Input: part model. Units: mm. Frame: model coordinates. Face numbers are marked on the shaded views. A direction names the side the tool comes from. Give positions to 0.01 mm unless a question says otherwise; leave off trailing zeros. Order: outer loops, then holes, each group sorted by start corner. A loop starts at its lowest first (then second) coordinate and runs counter-clockwise, first axis right, second up.
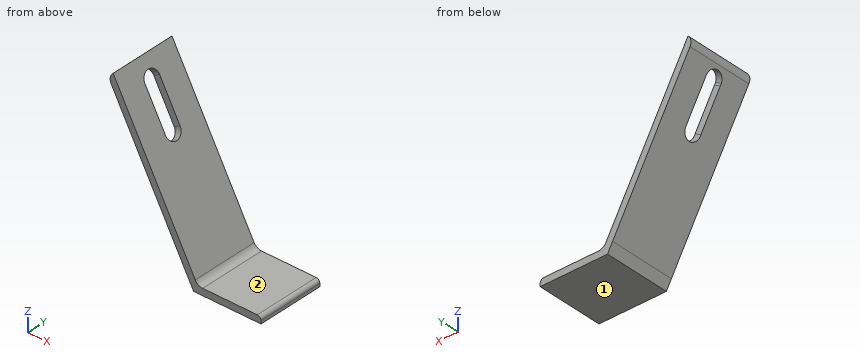
```python
from build123d import *

# Parameters (mm, degrees)
F1_DEPTH    = 40
F2_T1_DEPTH = 40
F2_T3_DEPTH = 64.4948974279
F3_T1_DEPTH = 50.8639610307
F5_DEPTH    = 25


# Not quite as in the source:
# - a fillet or chamfer that OpenCascade refuses, or shapes differently, is made with other operations: its cross-section is extruded or revolved along the edge and cut away or added
# - a feature names something its author has since deleted; it is built from what else it names


with BuildPart() as f1:
    # F0 (on Front) → F1 (new body)
    with BuildSketch(Plane.XZ):
        Polygon((-51.3135007212, 94.3231601012), (-3, 5.5145230071), (0, 0), (40, 0), (40, 4), (2.3775297152, 4), (-47.7997987259, 96.2346773752), align=None)
    extrude(amount=F1_DEPTH)

    # F2: fillet of radius 5 on 2 edges, made by hand

    # F2_s2 → F2_t1 (join)
    with BuildSketch(Plane.XZ):
        with BuildLine():
            ThreePointArc((5.3494418593, 4), (2.7947386439, 4.7019200239), (0.9573143652, 6.6106034076))
            Line((0.9573143652, 6.6106034076), (2.3775297152, 4))
            Line((2.3775297152, 4), (5.3494418593, 4))
        make_face()
    extrude(amount=F2_T1_DEPTH)

    # F2_s4 → F2_t3 (cut)
    with BuildSketch(Plane.XZ.offset(-12.2474487139)):
        with BuildLine():
            ThreePointArc((-47.7997987259, 96.2346773752), (-49.4935666702, 93.3361748844), (-48.9723797433, 90.019771603))
            Line((-48.9723797433, 90.019771603), (-51.3135007212, 94.3231601012))
            Line((-51.3135007212, 94.3231601012), (-47.7997987259, 96.2346773752))
        make_face()
    extrude(amount=F2_T3_DEPTH, mode=Mode.SUBTRACT)

    # F3: fillet of radius 2.1727922061 on 2 edges, made by hand

    # F3_s2 → F3_t1 (cut)
    with BuildSketch(Plane.XZ.offset(-5.4319805153)):
        with BuildLine():
            ThreePointArc((37.8272077939, 4), (39.3636038969, 3.3636038969), (40, 1.8272077939))
            Line((40, 1.8272077939), (40, 4))
            Line((40, 4), (37.8272077939, 4))
        make_face()
    extrude(amount=F3_T1_DEPTH, mode=Mode.SUBTRACT)

    # F4 (on face) → F5 (cut)
    with BuildSketch(Plane(origin=(3.5137019952, 0, 1.9115172739), x_dir=(0, 1, 0), z_dir=(0.8784254988, 0, 0.4778793185))):
        with BuildLine():
            Line((-15, 69.8649734259), (-15, 95.260605216))
            ThreePointArc((-15, 95.260605216), (-19.6685312037, 100.2496059614), (-24.9560513748, 95.9220844447))
            Line((-24.9560513748, 95.9220844447), (-24.9560513748, 94.5991259873))
            Line((-24.9560513748, 94.5991259873), (-24.9560513748, 70.5264526546))
            ThreePointArc((-24.9560513748, 70.5264526546), (-20.3314687963, 64.8759726805), (-15, 69.8649734259))
        make_face()
        with BuildLine():
            Line((-24.9560513748, 94.5991259873), (-24.9560513748, 95.9220844447))
            ThreePointArc((-24.9560513748, 95.9220844447), (-25, 95.260605216), (-24.9560513748, 94.5991259873))
        make_face()
    extrude(amount=-F5_DEPTH, mode=Mode.SUBTRACT)


solid = f1.part
```
1) First-contact query: P1, Ø8, axis at x = -28, y = -4, coming from the +Z side; P2, Ø12, axis at y = -27, z = 50, coming from the -X side (3 decimals); P3, Ø1, axis at y = -26, z = 12, coming from the -X side. Flat tips, straight axial feed; report the tip coordinate or a pass-through.
2) Cut plane D-D (x = 27.5). Return the cut outline in (y, z), then the cut area to 3 significant figures.
3) Line query: probe 1 along Z at (x, y) = (26.5, -22.5); probe 2 along X at (y, z) = (-24.5, 37); probe 3 along Z at (x, y) = (-11, -31.5). Output: solid intervals per line, ascending.
4) Reachability of the marked faces 1 and 2 from +Z, -Z, +X, -X, +Y, -Y: full face, straight path, thin tool, end or side. Return the list, or none.
5) Cut plane A-A (y = -12.5). Return the cut outline in (x, z).
6) Cut plane B-B (z = 78.5). Return the cut outline in (x, y).
7) Cut plane C-C (y = -19). Return the cut outline in (x, z).
Geometry says:
1. P1: stops at z = 67.19
1. P2: stops at x = -30.465
1. P3: stops at x = -6.8
2. outline: (-40, 0) - (0, 0) - (0, 4) - (-40, 4) - close
2. area: 160 mm2
3. probe 1: z = 0 to 4
3. probe 2: x = -20.13 to -15.58
3. probe 3: z = 20.22 to 28.59
4. face 1: -Z, +X, -X, +Y, -Y
4. face 2: +Z, +X, +Y, -Y
5. outline: (-48.97, 90.02) - (0, 0) - (40, 0) - (40, 1.83) arc R2.17 ccw to (37.83, 4) - (5.35, 4) arc R5 cw to (0.96, 6.61) - (-47.8, 96.23) arc R5 ccw to start
6. outline: (-42.71, -40) - (-38.15, -40) - (-38.15, -24.96) - (-42.71, -24.96) - close; (-42.71, -15) - (-38.15, -15) - (-38.15, 0) - (-42.71, 0) - close
7. outline: (-48.97, 90.02) - (-47.86, 87.98) - (-44.35, 89.89) - (-47.8, 96.23) arc R5 ccw to start; (-31.05, 57.07) - (0, 0) - (40, 0) - (40, 1.83) arc R2.17 ccw to (37.83, 4) - (5.35, 4) arc R5 cw to (0.96, 6.61) - (-27.53, 58.98) - close
